Work out the finished part from the listing and answer in its coordinate system (mm). A direction names the side the tool comes from. Round coordinates to 2 decimals unless told otherwise and drop trailing zeros. Write each loop counter-clockwise with the first axis right and the second up, starting at its lowest first coordinate (ties: lowest second). Pieces come first, ordered by that corner, then holes. Notation, with made-up numbers: (51, 28) -> (69, 28) arc R25 ccw to (69, 51) -> close; hole circle Ø8 at (-5.75, 82.25). An arc over 180 degrees is marked (long way). One line per item, written item: value.
```python
from build123d import *

# Parameters (mm, degrees)
SKETCH1_R           = 2
BOSS_EXTRUDE1_DEPTH = 1
SCALE1_SCALE        = 1.1


with BuildPart() as part:
    # Sketch1 → Boss-Extrude1 (new body)
    with BuildSketch(Plane.XY):
        with BuildLine():
            Line((-0.462098351, 6.089690496), (-1.629279619, 3.653142199))
            ThreePointArc((-1.629279619, 3.653142199), (-2.351141009, 3.236067977), (-2.970869602, 2.67842002))
            Line((-2.970869602, 2.67842002), (-5.648843585, 2.321299502))
            ThreePointArc((-5.648843585, 2.321299502), (-6.085555848, 1.977316958), (-5.934436072, 1.442336206))
            Line((-5.934436072, 1.442336206), (-3.977819784, -0.420653976))
            ThreePointArc((-3.977819784, -0.420653976), (-3.804226065, -1.236067977), (-3.465378009, -1.99778759))
            Line((-3.465378009, -1.99778759), (-3.953275684, -4.655048506))
            ThreePointArc((-3.953275684, -4.655048506), (-3.761080354, -5.176683001), (-3.205584845, -5.198277698))
            Line((-3.205584845, -5.198277698), (-0.829148209, -3.913120653))
            ThreePointArc((-0.829148209, -3.913120653), (0, -4), (0.829148209, -3.913120653))
            Line((0.829148209, -3.913120653), (3.205584845, -5.198277698))
            ThreePointArc((3.205584845, -5.198277698), (3.761080354, -5.176683001), (3.953275684, -4.655048506))
            Line((3.953275684, -4.655048506), (3.465378009, -1.99778759))
            ThreePointArc((3.465378009, -1.99778759), (3.804226065, -1.236067977), (3.977819784, -0.420653976))
            Line((3.977819784, -0.420653976), (5.934436072, 1.442336206))
            ThreePointArc((5.934436072, 1.442336206), (6.085555848, 1.977316958), (5.648843585, 2.321299502))
            Line((5.648843585, 2.321299502), (2.970869602, 2.67842002))
            ThreePointArc((2.970869602, 2.67842002), (2.351141009, 3.236067977), (1.629279619, 3.653142199))
            Line((1.629279619, 3.653142199), (0.462098351, 6.089690496))
            ThreePointArc((0.462098351, 6.089690496), (0, 6.398732088), (-0.462098351, 6.089690496))
        make_face()
        Circle(SKETCH1_R, mode=Mode.SUBTRACT)
    extrude(amount=BOSS_EXTRUDE1_DEPTH)


with BuildPart() as part_1:
    # Scale1: scaled about (0, 0, 0.5)
    add(part.part.scale(SCALE1_SCALE).moved(Location((0, 0, -0.05))))


solid = part_1.part
```
(1) A flat-ended cylindrical pin translates along its axis: pin 1 Ø2.5 at (x, y) = (0, 0) entering from +Z. Find the tip coordinate at first contact, or state that the pin passes through.
Reported:
pin 1: passes through
(2) For a pull along X with two mould halves and no side action, classify faces 4 (the face through (2.1, 0.66, 0.49)), 5 (the face through (-2.576, 3.567, 0.492)), 6 (the face through (1.16, 5.34, 0.49)) as pulls with the +X half, pulls with the -X half, needs draft (parallel to the pull), parting line crosses it, or undercut.
Reported:
face 4: undercut
face 5: pulls with the -X half
face 6: pulls with the +X half
(3) A tool of negligible diameter and unlimited length cuts with its end or side. For faces 1 (the face through (-4.189, -1.347, 0.492)), 2 (the face through (4.084, -3.68, 0.492)), 3 (the face through (2.2, -5, 0.5)), from which of +Z, -Z, +X, -X, +Y, -Y can it reach the whole face along a straight path? Write none if from no direction.
Reported:
face 1: +Z, -Z, -X
face 2: +Z, -Z, +X
face 3: +Z, -Z, -Y
(4) Find section C-C on y = 0.25. Give the vertices of the cut face in (x, z), plus the area to 3 significant figures.
Reported:
outline: (-5.12, -0.05) -> (-2.19, -0.05) -> (-2.19, 1.05) -> (-5.12, 1.05) -> close; (2.19, -0.05) -> (5.12, -0.05) -> (5.12, 1.05) -> (2.19, 1.05) -> close
area: 6.46 mm2
(5) Find section B-B on z = 0.1. Give the vertices of the cut face in (x, y), plus the area to 3 significant figures.
Reported:
outline: (-6.53, 1.59) -> (-4.38, -0.46) arc R4.4 ccw to (-3.81, -2.2) -> (-4.35, -5.12) arc R0.55 ccw to (-3.53, -5.72) -> (-0.91, -4.3) arc R4.4 ccw to (0.91, -4.3) -> (3.53, -5.72) arc R0.55 ccw to (4.35, -5.12) -> (3.81, -2.2) arc R4.4 ccw to (4.38, -0.46) -> (6.53, 1.59) arc R0.55 ccw to (6.21, 2.55) -> (3.27, 2.95) arc R4.4 ccw to (1.79, 4.02) -> (0.51, 6.7) arc R0.55 ccw to (-0.51, 6.7) -> (-1.79, 4.02) arc R4.4 ccw to (-3.27, 2.95) -> (-6.21, 2.55) arc R0.55 ccw to start; hole circle Ø4.4 at (0, 0)
area: 73.1 mm2
(6) Find section A-A on x = 0. Give the vertices of the cut face in (y, z), plus the area to 3 significant figures.
Reported:
outline: (-4.4, -0.05) -> (-2.2, -0.05) -> (-2.2, 1.05) -> (-4.4, 1.05) -> close; (2.2, -0.05) -> (7.04, -0.05) -> (7.04, 1.05) -> (2.2, 1.05) -> close
area: 7.74 mm2
(7) Consider probe 1 along X at (y, z) = (-0.75, 0.2); probe 2 along Y at (x, z) = (1, 0.05); probe 3 along X at (y, z) = (-0.25, 0.9). Determine where each line is inside the solid, lowest interval first.
Reported:
probe 1: x = -4.34 to -2.07, 2.07 to 4.34
probe 2: y = -4.35 to -1.96, 1.96 to 5.67
probe 3: x = -4.6 to -2.19, 2.19 to 4.6
(8) Find section D-D on x = -2.75. Give the vertices of the cut face in (y, z).
Reported:
outline: (-5.3, -0.05) -> (3.43, -0.05) -> (3.43, 1.05) -> (-5.3, 1.05) -> close
